Drawing for the job (mm, zero at the part's lowest x, y, z). A direction names the side the tool comes from. Coordinates: 2 decimals unless noted, no trailing zeros. Write each loop counter-clockwise with the first axis right and the second up, starting at its lowest first coordinate (ties: lowest second). Pieces come first, ordered by that corner, then holes. Notation, with made-up numbers: (60.25, 65) -> (64.25, 65) arc R21 cw to (64.25, 72) -> close; hole circle Ø8 at (32.5, 19.25). An arc over 180 degrees is marked (long way). Write item = value, one per line. Start each with the question number.
Q1. Band-saw the part on D-D, the plane z = 8.5. List the corners of the cut face in (x, y), plus the area to 3 significant figures.
Q2. Probe line 1 (X direction, y = 3.5, z = 8.75); line 2 (Y direction, x = 31.5, z = 8.5); line 3 (Z direction, x = 16, y = 9.25) (1 decimal). List the from-to ranges inside material, lowest first.
Q3. Tool access for the marked faces 1, 2 and 3: list every direction of +Z, -Z, +X, -X, +Y, -Y with a clear straight run to the whole face (end or side of a thin tool).
Q4. Pin check, flat tip, straight feed: P1, Ø3, axis at x = 29, y = 6, coming from the +Z side. Stop position of the tip, or through.
Q5. Band-saw the part on C-C, the plane y = 1.75. List the corners of the cut face in (x, z), plus the area to 3 significant figures.
Q6. Band-saw the part on B-B, the plane x = 30. List the corners of the cut face in (y, z).
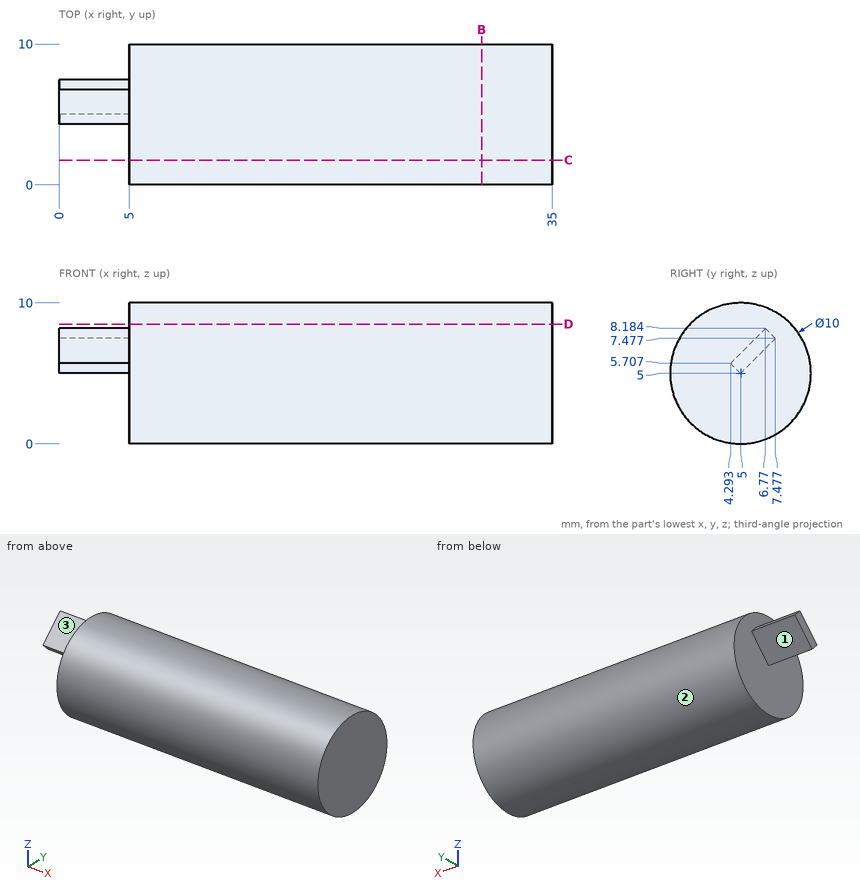
Ans:
q1.outline = (5, 1.43) -> (35, 1.43) -> (35, 8.57) -> (5, 8.57) -> close
q1.area = 214 mm2
q2.line_1 = 5 to 35
q2.line_2 = 1.43 to 8.57
q2.line_3 = 2.4 to 7.6
q3.face_1 = -Z, -X, +Y
q3.face_2 = +X, -X
q3.face_3 = +Z, -X, -Y
q4.P1 = 10
q5.outline = (5, 1.2) -> (35, 1.2) -> (35, 8.8) -> (5, 8.8) -> close
q5.area = 228 mm2
q6.outline = circle Ø10 at (5, 5)
